```python
from build123d import *
from build123d.topology import SkipClean

# Parameters (mm, degrees)
SKETCH1_R           = 7.5
SKETCH1_R_2         = 5
BOSS_EXTRUDE1_DEPTH = 99
SKETCH2_R           = 10
BOSS_EXTRUDE2_DEPTH = 17.5
SKETCH3_R           = 10
SKETCH3_R_2         = 7.5
BOSS_EXTRUDE3_DEPTH = 17.5
SKETCH4_R           = 10
SKETCH4_R_2         = 7.5
BOSS_EXTRUDE4_DEPTH = 17.5
SKETCH5_R           = 10
SKETCH5_R_2         = 7.5
BOSS_EXTRUDE5_DEPTH = 17.5
SKETCH6_R           = 10
SKETCH6_R_2         = 7.5
BOSS_EXTRUDE6_DEPTH = 17.5
SKETCH9_R           = 7.5
SKETCH9_R_2         = 5
BOSS_EXTRUDE7_DEPTH = 0.5
SKETCH10_R          = 5
CUT_EXTRUDE1_DEPTH  = 84.210576251


with BuildPart() as part:
    # Sketch1 → Boss-Extrude1 (new body)
    with BuildSketch(Plane.XY):
        Circle(SKETCH1_R)
        Circle(SKETCH1_R_2, mode=Mode.SUBTRACT)
    extrude(amount=BOSS_EXTRUDE1_DEPTH)

    # Sketch2 → Boss-Extrude2 (add)
    with BuildSketch(Plane(origin=(0, 0, 0), x_dir=(-1, 0, 0), z_dir=(0, 0, -1))):
        Circle(SKETCH2_R)
    extrude(amount=-BOSS_EXTRUDE2_DEPTH)

    # Sketch3 → Boss-Extrude3 (add)
    with BuildSketch(Plane.XY.offset(20.5)):
        Circle(SKETCH3_R)
        Circle(SKETCH3_R_2, mode=Mode.SUBTRACT)
    extrude(amount=BOSS_EXTRUDE3_DEPTH)

    # Sketch4 → Boss-Extrude4 (add)
    with BuildSketch(Plane.XY.offset(41)):
        Circle(SKETCH4_R)
        Circle(SKETCH4_R_2, mode=Mode.SUBTRACT)
    extrude(amount=BOSS_EXTRUDE4_DEPTH)

    # Sketch5 → Boss-Extrude5 (add)
    with BuildSketch(Plane.XY.offset(61.5)):
        Circle(SKETCH5_R)
        Circle(SKETCH5_R_2, mode=Mode.SUBTRACT)
    extrude(amount=BOSS_EXTRUDE5_DEPTH)

    # Sketch6 → Boss-Extrude6 (add)
    with BuildSketch(Plane.XY.offset(82)):
        Circle(SKETCH6_R)
        Circle(SKETCH6_R_2, mode=Mode.SUBTRACT)
    extrude(amount=BOSS_EXTRUDE6_DEPTH)

    # Sketch9 → Boss-Extrude7 (add)
    with BuildSketch(Plane.XY.offset(99)):
        Circle(SKETCH9_R)
        with Locations(Location((0, 0, 0), (0, 0, 180))):
            Circle(SKETCH9_R_2, mode=Mode.SUBTRACT)
    extrude(amount=BOSS_EXTRUDE7_DEPTH)

    # Sketch10 → Cut-Extrude1 (cut, through all)
    with SkipClean():  # the faces are left unmerged after this step: merging them gives an invalid solid
        with BuildSketch(Plane.XY.offset(17.5)):
            Circle(SKETCH10_R)
        extrude(amount=-CUT_EXTRUDE1_DEPTH, mode=Mode.SUBTRACT)
    add(part.part.scale(1), mode=Mode.REPLACE)  # the faces are merged on a copy


solid = part.part
```
Source: CAD feature listing. Evaluate the final solid. Frame: model axes, mm. A direction names the side the tool comes from. Give positions to 0.01 mm unless a question says otherwise; leave off trailing zeros. Order: outer loops, then holes, each group sorted by start corner. A loop starts at its lowest first (then second) coordinate and runs counter-clockwise, first axis right, second up. Notation, with made-up numbers: (23.25, 37.5) -> (69.25, 37.5) arc R23 ccw to (69.25, 60.5) -> close; hole circle Ø3 at (72, 6.5). An arc over 180 degrees is marked (long way). Use a Markdown table: item, result.
Q1. Section C-C (z = 24.5). Return the cut outline in (x, y).
A:
| item | result |
|---|---|
| outline | circle Ø20 at (0, 0); hole circle Ø10 at (0, 0) |
Q2. First-contact query: P1, Ø6, axis at x = -3.5, z = 83.5, coming from the +Y side; P2, Ø1.5, axis at x = 5, z = 89, coming from the +Y side; P3, Ø3, axis at y = 6.5, z = 65, coming from the -X side; P4, Ø6, axis at x = 0, y = 0, coming from the -Z side. Flat tips, straight axial feed; report the tip coordinate or a pass-through.
A:
| item | result |
|---|---|
| P1 | y = 9.99 |
| P2 | y = 9.05 |
| P3 | x = -8.66 |
| P4 | through |
Q3. Pull-direction query (Z, two-part tool) for faces 1 (the face through (2, 5, 99.5)), 2 (the face through (4, 7, 58.5)), 3 (the face through (-2.17, -9.76, 90.63)); classes: +Z half, -Z half, draft (parallel to the pull), parting line (faces both ways), or undercut.
A:
| item | result |
|---|---|
| face 1 | +Z half |
| face 2 | undercut |
| face 3 | draft |
Q4. Access query for faces 4 (the face through (4, 7, 41)), 5 (the face through (-2.17, -9.76, 49.63)). Directions: +Z, -Z, +X, -X, +Y, -Y. A direction counts if a zero-diameter tool reaches every point of the face in a straight line with its end or side. Return the directions, or none.
A:
| item | result |
|---|---|
| face 4 | none |
| face 5 | +Z, -Z |
Q5. Material intervals for line 1 (Z direction, x = 2.5, y = -9); line 2 (Y direction, x = 0, z = 39.5); line 3 (Y direction, x = 0, z = 44), sorted ascending. Write a range as [from, to].
A:
| item | result |
|---|---|
| line 1 | [0, 17.5], [20.5, 38], [41, 58.5], [61.5, 79], [82, 99.5] |
| line 2 | [-7.5, -5], [5, 7.5] |
| line 3 | [-10, -5], [5, 10] |
Q6. Section B-B (x = -8.5). Return the cut outline in (y, z), and give its area (3 significant figures).
A:
| item | result |
|---|---|
| outline | (-5.27, 0) -> (5.27, 0) -> (5.27, 17.5) -> (-5.27, 17.5) -> close; (-5.27, 20.5) -> (5.27, 20.5) -> (5.27, 38) -> (-5.27, 38) -> close; (-5.27, 41) -> (5.27, 41) -> (5.27, 58.5) -> (-5.27, 58.5) -> close; (-5.27, 61.5) -> (5.27, 61.5) -> (5.27, 79) -> (-5.27, 79) -> close; (-5.27, 82) -> (5.27, 82) -> (5.27, 99.5) -> (-5.27, 99.5) -> close |
| area | 922 mm^2 |
